Read the model definition and answer for the solid it produces. Units are mm, in the model's axes. A direction names the side the tool comes from. Give positions to 0.01 mm unless a question says otherwise; leave off trailing zeros. Loops run counter-clockwise (first coordinate to the right, second up) from the corner with the lowest first, then second, coordinate; pieces in that order, holes last. Notation, with made-up numbers: (-25.5, 20.25) -> (-16.5, 20.25) arc R5 cw to (-16.5, 28.25) -> close; hole circle Ø11 at (36.5, 79.5). An arc over 180 degrees is marked (long way). Return JSON: item names as keys, results as strings. Group by question number.
from build123d import *

# Parameters (mm, degrees)
SKETCH1_W           = 100
SKETCH1_H           = 65.6
BOSS_EXTRUDE1_DEPTH = 2
SKETCH2_W           = 3.96828804
SKETCH2_H           = 11.261454498
BOSS_EXTRUDE2_DEPTH = 2
SKETCH3_W           = 2
SKETCH3_H           = 2
BOSS_EXTRUDE3_DEPTH = 10


with BuildPart() as part:
    # Sketch1 → Boss-Extrude1 (new body)
    with BuildSketch(Plane.XY):
        Rectangle(SKETCH1_W, SKETCH1_H)
    extrude(amount=BOSS_EXTRUDE1_DEPTH)

    # Sketch2 → Boss-Extrude2 (add)
    with BuildSketch(Plane(origin=(50, 0, 0), x_dir=(0, 0, -1), z_dir=(1, 0, 0))):
        with Locations((-1, 0)):
            Rectangle(SKETCH2_W, SKETCH2_H)
    extrude(amount=BOSS_EXTRUDE2_DEPTH)

    # Sketch3 → Boss-Extrude3 (add)
    with BuildSketch(Plane(origin=(52, 0, 0), x_dir=(0, 0, -1), z_dir=(1, 0, 0))):
        with Locations((-1, 0)):
            Rectangle(SKETCH3_W, SKETCH3_H)
    extrude(amount=BOSS_EXTRUDE3_DEPTH)


solid = part.part
1. Section C-C on x = 33 is taken. Determine the outline of the cut face in (y, z).
2. Which of the six approach directions +Z, -Z, +X, -X, +Y, -Y give full straight-line access (tool end or side, diameter ignored) to faces 1 (the flat face through (51, -5.631, 1)), 2 (the flat face through (57, 1, 1)), 3 (the flat face through (57, 0, 0)), 4 (the flat face through (57, 0, 2))?
3. Section A-A on z = 1.3 is taken. Determine the outline of the cut face in (x, y), then the cut area to 3 significant figures.
4. Straight lines are drawn through the part: line 1 (X direction, y = -21, z = 0.9); line 2 (Z direction, x = 33.5, y = -24); line 3 (X direction, y = -4, z = -0.45). For each, find the intervals that lie inside material, in ascending order. Write a range as from..to.
5. Flat-ended cylindrical pins translate along their axes: pin 1 Ø6 at (x, y) = (18.5, -12) entering from +Z; pin 2 Ø1 at (x, z) = (51, 0) entering from +Y; pin 3 Ø0.6 at (y, z) = (22.5, 1) entering from +X. Find the tip coordinate at first contact, or state that the pin passes through.
6. Section B-B on y = 2.5 is taken. Determine the outline of the cut face in (x, z), then the cut area to 3 significant figures.
7. Section D-D on y = 24 is taken. Determine the outline of the cut face in (x, z).
Completed:
{
 "1": {"outline": "(-32.8, 0) -> (32.8, 0) -> (32.8, 2) -> (-32.8, 2) -> close"},
 "2": {"face 1": "+Z, -Z, +X, -Y", "face 2": "+Z, -Z, +X, +Y", "face 3": "-Z, +X, +Y, -Y", "face 4": "+Z, +X, +Y, -Y"},
 "3": {"outline": "(-50, -32.8) -> (50, -32.8) -> (50, -5.63) -> (52, -5.63) -> (52, -1) -> (62, -1) -> (62, 1) -> (52, 1) -> (52, 5.63) -> (50, 5.63) -> (50, 32.8) -> (-50, 32.8) -> close", "area": "6,600 mm²"},
 "4": {"line 1": "x = -50..50", "line 2": "z = 0..2", "line 3": "x = 50..52"},
 "5": {"pin 1": "stops at z = 2", "pin 2": "stops at y = 5.63", "pin 3": "stops at x = 50"},
 "6": {"outline": "(-50, 0) -> (50, 0) -> (50, -0.98) -> (52, -0.98) -> (52, 2.98) -> (50, 2.98) -> (50, 2) -> (-50, 2) -> close", "area": "208 mm²"},
 "7": {"outline": "(-50, 0) -> (50, 0) -> (50, 2) -> (-50, 2) -> close"}
}
